Can you work these out from the model? Positions are in its coordinate system, mm. A direction names the side the tool comes from. Round coordinates to 2 decimals unless told otherwise and drop trailing zeros. Write each question's results on one line, items separated by ' | '.
from build123d import *

# Parameters (mm, degrees)
F1_DEPTH = 2.999994
F2_R     = 1.65
F2_R_2   = 2.705
F2_R_3   = 2.11
F2_W     = 3.0734
F2_H     = 9.398
F3_DEPTH = 3.000994
F5_DEPTH = 3.000994


with BuildPart() as f1:
    # F0 (on Top) → F1 (new body)
    with BuildSketch(Plane.XY):
        with BuildLine():
            Line((-17.25041, -77.999971), (17.25041, -77.999971))
            ThreePointArc((17.25041, -77.999971), (20.785937, -76.535508), (22.2504, -72.999981))
            Line((22.2504, -72.999981), (22.2504, 72.999981))
            ThreePointArc((22.2504, 72.999981), (20.785937, 76.535508), (17.25041, 77.999971))
            Line((17.25041, 77.999971), (-17.25041, 77.999971))
            ThreePointArc((-17.25041, 77.999971), (-20.785937, 76.535508), (-22.2504, 72.999981))
            Line((-22.2504, 72.999981), (-22.2504, -72.999981))
            ThreePointArc((-22.2504, -72.999981), (-20.785937, -76.535508), (-17.25041, -77.999971))
        make_face()
    extrude(amount=-F1_DEPTH)

    # F2 (on face) → F3 (cut, through all)
    with BuildSketch(Plane.XY):
        with Locations((-9.99998, -67.999991)):
            Circle(F2_R)
        with Locations((-12.7004, -58.019971)):
            Circle(F2_R_2)
        with Locations((-14.5004, -7.399971)):
            Circle(F2_R_3)
        with Locations((-10.0004, 40.501189)):
            Circle(F2_R)
        with Locations((-14.5004, 49.600029)):
            Circle(F2_R_3)
        with BuildLine():
            ThreePointArc((0, -13.374971), (-2.7054, -16.079971), (0, -18.784971))
            Line((0, -18.784971), (0, -13.374971))
        make_face()
        with BuildLine():
            Line((0, -13.374971), (0, -18.784971))
            ThreePointArc((0, -18.784971), (1.912465, -17.992553), (2.7046, -16.079971))
            ThreePointArc((2.7046, -16.079971), (1.912465, -14.167389), (0, -13.374971))
        make_face()
        with Locations((9.99998, -67.999991)):
            Circle(F2_R)
        with Locations((12.7004, -58.019971)):
            Circle(F2_R_2)
        with Locations((14.5004, -7.399971)):
            Circle(F2_R_3)
        with Locations((10.0004, 40.501189)):
            Circle(F2_R)
        with Locations((14.5004, 49.600029)):
            Circle(F2_R_3)
        with Locations((-15.9637, -47.900971)):
            Rectangle(F2_W, F2_H)
        with Locations((-15.9637, 28.299029)):
            Rectangle(F2_W, F2_H)
        with Locations((15.9637, 28.299029)):
            Rectangle(F2_W, F2_H)
        with Locations((15.9637, -47.900971)):
            Rectangle(F2_W, F2_H)
    extrude(amount=-F3_DEPTH, mode=Mode.SUBTRACT)

    # F4 (on face) → F5 (cut, through all)
    with BuildSketch(Plane.XY):
        with BuildLine():
            ThreePointArc((-22.2504, 69.297931), (-20.785937, 72.833458), (-17.25041, 74.297921))
            Line((-17.25041, 74.297921), (17.25041, 74.297921))
            ThreePointArc((17.25041, 74.297921), (20.785937, 72.833458), (22.2504, 69.297931))
            Line((22.2504, 69.297931), (22.2504, 72.999981))
            ThreePointArc((22.2504, 72.999981), (20.785937, 76.535508), (17.25041, 77.999971))
            Line((17.25041, 77.999971), (-17.25041, 77.999971))
            ThreePointArc((-17.25041, 77.999971), (-20.785937, 76.535508), (-22.2504, 72.999981))
            Line((-22.2504, 72.999981), (-22.2504, 69.297931))
        make_face()
    extrude(amount=-F5_DEPTH, mode=Mode.SUBTRACT)


solid = f1.part
1. If we section it at A-A (z = -1.35): State how many separate pieces and enclosed holes the cut face has, then the cut area to 3 significant figures.
Final values:
separate pieces: 1 | enclosed holes: 15 | area: 6,480 mm2
2. On a 3-axis mill with a long thin cutter (end or side, diameter ignored), from which of +Z, -Z, +X, -X, +Y, -Y can I reach the whole of each face in a straight line? I mean faces 4 (the face through (14.427, 28, -1)), 5 (the face through (-20.825, 72.794, -1.479)). Say none if no direction works.
Final values:
face 4: +Z, -Z | face 5: +Z, -Z, -X, +Y
3. Will this pin go through, and if not, where does the flat tip stop? pin 1 (3 mm diameter, centred on x = 10, y = -68, fed in from +Z).
Final values:
pin 1: through
4. Please list where these lines run through material, in increasing order: line 1 (Y direction, x = 17, z = -2.65); line 2 (Y direction, x = -15.5, z = -2.55); line 3 (Y direction, x = -15, z = -0.4). Write a range as from..to.
Final values:
line 1: -78..-52.6, -43.2..23.6, 33..74.3 | line 2: -78..-52.6, -43.2..-9.26, -5.54..23.6, 33..47.74, 51.46..74.3 | line 3: -78..-59.44, -56.6..-52.6, -43.2..-9.45, -5.35..23.6, 33..47.55, 51.65..74.3
5. We'd pull the mould along Y, two halves only. Please class faces 1 (the face through (20.75, -76.57, -1.48)), 2 (the face through (-16, -43.202, -1)), 3 (the face through (-22.25, -1, -1)): pulls with the +Y half, pulls with the -Y half, needs draft (parallel to the pull), parting line crosses it, or undercut.
Final values:
face 1: pulls with the -Y half | face 2: undercut | face 3: needs draft
